Could you check a few things on this model? Use its own coordinates, in mm. Coordinates: 2 decimals unless noted, no trailing zeros. Order: outer loops, then holes, each group sorted by start corner. A loop starts at its lowest first (then second) coordinate and runs counter-clockwise, first axis right, second up. Notation, with made-up numbers: (50, 52.25) -> (90, 52.25) arc R16 ccw to (90, 68.25) -> close; hole circle Ø4 at (-24.75, -28.75). An arc over 180 degrees is marked (long way). Use a Markdown table: item, result. Add a question column.
1) If I drill on L1, parallel to Y at x = -143.5, z = 275.5; L2, parallel to X at y = -35.5, z = 232; L3, parallel to X at y = -59.5, z = 229.5, over which ranges is the centre line in solid material (lowest first)? Write a range as [from, to].
2) Will this pin go through, and if not, where does the flat tip stop? pin 1 Ø8 at (x, z) = (85, 91.5) entering from -Y.
3) If we section it at B-B (x = -57.5): Write out the boundary of the cut face in (y, z).
4) If we section it at C-C (y = -35): Write out the boundary of the cut face in (x, z).
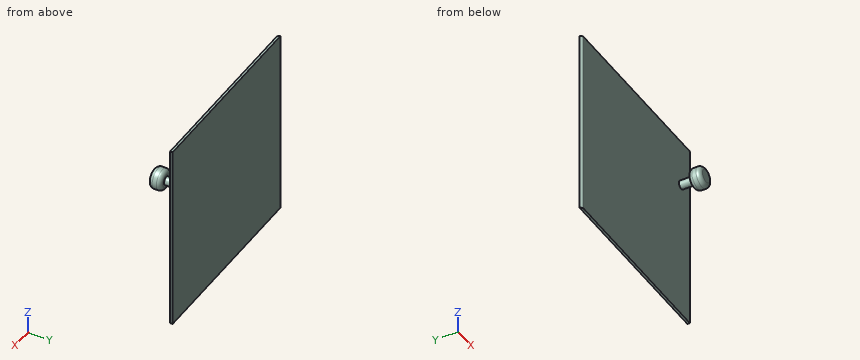
```python
from build123d import *

# Parameters (mm, degrees)
F0_W     = 571.5
F0_H     = 584.2
F1_DEPTH = 7.62
F2_R     = 7.61999
F3_R     = 12.7
F4_DEPTH = 38.1
F5_R     = 31.75
F5_R_2   = 12.7
F6_DEPTH = 38.1
F7_R     = 12.7


# Not quite as in the source:
# - a fillet or chamfer is up to 0.001 mm smaller than in the source, because OpenCascade refuses the exact size


with BuildPart() as f1:
    # F0 (on Front) → F1 (new body)
    with BuildSketch(Plane.XZ):
        with Locations((-17.7775520504, 93.1158526728)):
            Rectangle(F0_W, F0_H)
    extrude(amount=F1_DEPTH)

    # F2 (radius 7.62 in the source; OpenCascade refuses exactly that, so slightly less here)
    f2_edges = [f1.edges().sort_by_distance(p)[0] for p in [
        (-303.527552, -7.62, 93.115853),
    ]]
    fillet(f2_edges, radius=F2_R)

    # F3 (on face) → F4 (join)
    with BuildSketch(Plane.XZ.offset(7.62)):
        with Locations((222.1034169197, 238.7578934431)):
            Circle(F3_R)
    extrude(amount=F4_DEPTH)

    # F5 (on face) → F6 (join)
    with BuildSketch(Plane.XZ.offset(45.72)):
        with Locations((222.1034169197, 238.7578934431)):
            Circle(F5_R)
        with Locations((222.1034169197, 238.7578934431)):
            Circle(F5_R_2, mode=Mode.SUBTRACT)
        with Locations((222.1034169197, 238.7578934431)):
            Circle(F5_R_2)
    extrude(amount=F6_DEPTH)

    # F7
    f7_edges = [f1.edges().sort_by_distance(p)[0] for p in [
        (190.353417, -83.82, 238.757893),
        (190.353417, -45.72, 238.757893),
    ]]
    fillet(f7_edges, radius=F7_R)


solid = f1.part
```
Answer sheet:
| question | item | result |
|---|---|---|
| 1 | L1 | [-7.62, 0] |
| 1 | L2 | [211.35, 232.86] |
| 1 | L3 | [191.73, 252.47] |
| 2 | pin 1 | y = -7.62 |
| 3 | outline | (-7.62, -198.98) -> (0, -198.98) -> (0, 385.22) -> (-7.62, 385.22) -> close |
| 4 | outline | circle Ø25.4 at (222.1, 238.76) |
